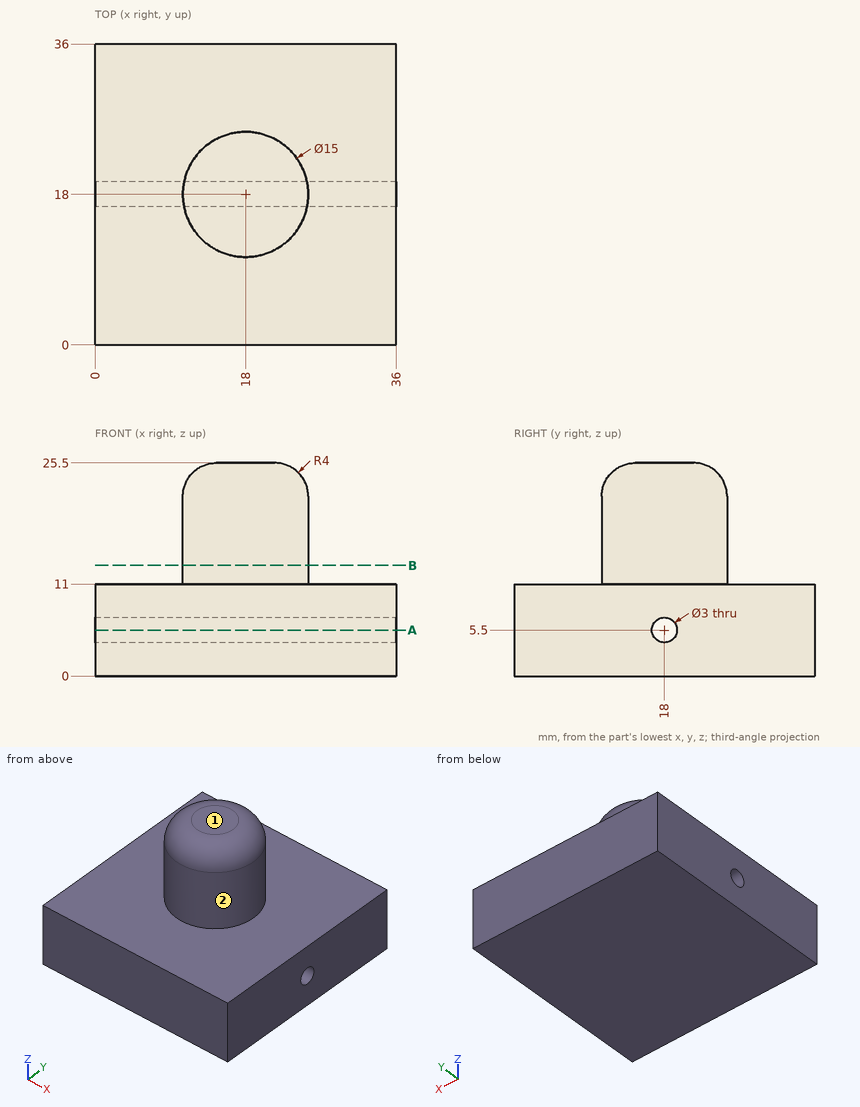
The drawing under review shows one solid part. Ordinate dimensions are in mm from its lowest x, y, z. A direction names the side the tool comes from. Round coordinates to 2 decimals unless told otherwise and drop trailing zeros. Loops run counter-clockwise (first coordinate to the right, second up) from the corner with the lowest first, then second, coordinate; pieces in that order, holes last. Notation, with made-up numbers: (13.5, 88.25) - (56.5, 88.25) arc R17 cw to (56.5, 110.25) - close; hole circle Ø10 at (71.25, 10.25). An arc over 180 degrees is marked (long way). Use a Markdown table: item, result. Add a question column.
Q1. Machinability: for the marked faces 1 and 2, which of the approach directions +Z, -Z, +X, -X, +Y, -Y give a long, thin tool a straight path to every point of the face, cutting with its end or side? Answer none if there is none.
Q2. Add section A-A (z = 5.5). State the section outline as (x, y) points.
Q3. Add section B-B (z = 13.25). State the section outline as (x, y) points.
Q4. Insertion check: pin 1 Ø5 at (x, z) = (15.5, 16.5) entering from +Y; pin 2 Ø8 at (x, z) = (16, 15.5) entering from -Y; pin 3 Ø6 at (y, z) = (25.5, 15.5) entering from +X; pin 4 Ø2.5 at (y, z) = (18, 5.5) entering from -X. Each pin has a flat end and moves straight along its axis. Give the tip position at first contact, or say it passes through.
Q5. For probe 1 along Y at (x, z) = (12.5, 5.5); probe 2 along Z at (x, y) = (22, 33); probe 3 along Y at (x, z) = (18, 6.5), list the stretches that pass through material, from the lowest coordinate up.
Worked answers:
| question | item | result |
|---|---|---|
| 1 | face 1 | +Z, +X, -X, +Y, -Y |
| 1 | face 2 | +Z |
| 2 | outline | (0, 0) - (36, 0) - (36, 16.5) - (0, 16.5) - close; (0, 19.5) - (36, 19.5) - (36, 36) - (0, 36) - close |
| 3 | outline | circle Ø15 at (18, 18) |
| 4 | pin 1 | y = 25.5 |
| 4 | pin 2 | y = 10.5 |
| 4 | pin 3 | x = 24 |
| 4 | pin 4 | through |
| 5 | probe 1 | 0 to 16.5, 19.5 to 36 |
| 5 | probe 2 | 0 to 11 |
| 5 | probe 3 | 0 to 16.88, 19.12 to 36 |
